from build123d import *

# Parameters (mm, degrees)
F2_DEPTH = 2.15
F3_R     = 0.5


with BuildPart() as f1:
    # F0 (on Front) → F1 (revolve)
    with BuildSketch(Plane.XZ):
        with BuildLine():
            Line((-2.15, 0), (-2.15, 5.8685603004))
            ThreePointArc((-2.15, 5.8685603004), (-5.9924786661, 1.7755842522), (-5, -3.75))
            Line((-5, -3.75), (0, -3.75))
            Line((0, -3.75), (0, 0))
            Line((0, 0), (-2.15, 0))
        make_face()
        with BuildLine():
            Line((0, 0), (0, 6.25))
            ThreePointArc((0, 6.25), (-1.0917870951, 6.153901278), (-2.15, 5.8685603004))
            Line((-2.15, 5.8685603004), (-2.15, 0))
            Line((-2.15, 0), (0, 0))
        make_face()
    revolve(axis=Axis((0, 0, 1.25), (0, 0, -1)))

    # F0 (on Front) → F2 (join, symmetric)
    with BuildSketch(Plane.XZ):
        with BuildLine():
            Line((0, 0), (0, 6.25))
            ThreePointArc((0, 6.25), (-1.0917870951, 6.153901278), (-2.15, 5.8685603004))
            Line((-2.15, 5.8685603004), (-2.15, 0))
            Line((-2.15, 0), (0, 0))
        make_face()
        with BuildLine():
            ThreePointArc((-2.15, 5.8685603004), (-1.0917870951, 6.153901278), (0, 6.25))
            Line((0, 6.25), (0, 0))
            Line((0, 0), (2.15, 0))
            Line((2.15, 0), (2.15, 13))
            Line((2.15, 13), (-2.15, 13))
            Line((-2.15, 13), (-2.15, 5.8685603004))
        make_face()
    extrude(amount=F2_DEPTH, both=True)

    # F3
    f3_edges = [f1.edges().sort_by_distance(p)[0] for p in [
        (-2.15, -2.15, 9.23027),
        (-2.15, 2.15, 9.23027),
        (2.15, -2.15, 9.23027),
        (2.15, 2.15, 9.23027),
    ]]
    fillet(f3_edges, radius=F3_R)


solid = f1.part
Work out the finished part from the listing and answer in its coordinate system (mm). Give positions to 0.01 mm unless a question says otherwise; leave off trailing zeros. Loops run counter-clockwise (first coordinate to the right, second up) from the corner with the lowest first, then second, coordinate; pieces in that order, holes last. Notation, with made-up numbers: (6, 46) - (45, 46) arc R33 cw to (45, 85) - close; hole circle Ø8 at (2.25, 47). An arc over 180 degrees is marked (long way). Answer in a Markdown table with one row per item. Add a question column.
Q1. The part is cut by section A-A (z = 7). Determine the outline of the cut face in (x, y), and give its area (3 significant figures).
Q2. Each of these flat-tipped pins is pushed along its axis until it touches: P1, Ø5, axis at x = 3.5, z = 5.5, coming from the -Y side; P2, Ø1.6, axis at x = 1, z = 8, coming from the -Y side; P3, Ø3, axis at y = 2, z = 4, coming from the +X side. Where does it stop, or does it pass through?
Q3. The part is cut by section C-C (y = -1.25). Determine the outline of the cut face in (x, z).
Q4. Consider line 1 along Y through (x, z) = (1, 9.5); line 2 along Z through (x, y) = (2.25, -1.5). Determine where each line is inside the solid, lowest interval first.
Q5. The part is cut by section B-B (x = 0). Determine the outline of the cut face in (y, z).
Q6. The part is cut by section D-D (z = 1.75). Determine the outline of the cut face in (x, y).
Solution:
| question | item | result |
|---|---|---|
| 1 | outline | (-2.15, -1.65) arc R0.5 ccw to (-1.65, -2.15) - (1.65, -2.15) arc R0.5 ccw to (2.15, -1.65) - (2.15, 1.65) arc R0.5 ccw to (1.65, 2.15) - (-1.65, 2.15) arc R0.5 ccw to (-2.15, 1.65) - close |
| 1 | area | 18.3 mm² |
| 2 | P1 | stops at y = -4.79 |
| 2 | P2 | stops at y = -2.15 |
| 2 | P3 | stops at x = 5.5 |
| 3 | outline | (-4.84, -3.75) - (4.84, -3.75) arc R6.12 ccw to (2.15, 5.73) - (2.15, 13) - (-2.15, 13) - (-2.15, 5.73) arc R6.12 ccw to start |
| 4 | line 1 | y = -2.15 to 2.15 |
| 4 | line 2 | z = -3.75 to 5.63 |
| 5 | outline | (-5, -3.75) - (5, -3.75) arc R6.25 ccw to (2.15, 5.87) - (2.15, 13) - (-2.15, 13) - (-2.15, 5.87) arc R6.25 ccw to start |
| 6 | outline | circle Ø12 at (0, 0) |
